```python
from build123d import *

# Parameters (mm, degrees)
BOSS_EXTRUDE1_DEPTH         = 40
TAP_DRILL_FOR_M6X1_0_TAP1_D = 5
TAP_DRILL_FOR_M6X1_0_TAP2_D = 5


with BuildPart() as part:
    # Sketch1 → Boss-Extrude1 (new body)
    with BuildSketch(Plane.XY):
        Polygon((0, 0), (0, -30), (32, -30), (32, -28), (2, -28), (2, 0), align=None)
    extrude(amount=BOSS_EXTRUDE1_DEPTH)

    # Tap Drill for M6x1.0 Tap1 (through all)
    with Locations(Plane(origin=(0, -28, 0), x_dir=(1, 0, 0), z_dir=(0, 1, 0))):
        with Locations((14.5, -7.5), (14.5, -32.5)):
            Hole(TAP_DRILL_FOR_M6X1_0_TAP1_D / 2)

    # Tap Drill for M6x1.0 Tap2 (through all)
    with Locations(Plane(origin=(2, 0, 0), x_dir=(0, 0, -1), z_dir=(1, 0, 0))):
        with Locations((-32, -14), (-8, -14)):
            Hole(TAP_DRILL_FOR_M6X1_0_TAP2_D / 2)


solid = part.part
```
Here's how the part is built. I have some questions about the finished solid (model axes, mm). A direction names the side the tool comes from. Round coordinates to 2 decimals unless told otherwise and drop trailing zeros. Order: outer loops, then holes, each group sorted by start corner. A loop starts at its lowest first (then second) coordinate and runs counter-clockwise, first axis right, second up. Notation, with made-up numbers: (29.25, 29.25) -> (59.25, 29.25) arc R17 ccw to (59.25, 38.25) -> close; hole circle Ø9 at (-12.75, -3). An arc over 180 degrees is marked (long way). Use a Markdown table: item, result. Add a question column.
(1) If we mould it in two halves opening along Z, with no side actions, what happens to faces 3 (the face through (17, -28, 20)), 4 (the face through (16.5, -29, 9)), 5 (the face through (8.8, -28.3, 40))? For each: released by +Z, released by -Z, zero draft, split by the parting line, or undercut.
(2) Suppose I cut it at D-D, the plane z = 3. Please give me the cut outline in (x, y), and give its area (3 significant figures).
(3) For faces 1 (the face through (16.34, -29.01, 30.81)), 2 (the face through (2, -14, 20)), which set-ups out of +Z, -Z, +X, -X, +Y, -Y let a thin tool reach every point of the face, with its end or its side?
(4) Suppose I cut it at A-A, the plane y = -14. Please give me the cut outline in (x, z).
(5) Suppose I cut it at C-C, the plane z = 32. Please give me the cut outline in (x, y).
(6) For pin 1 Ø1.5 at (y, z) = (-16.5, 10) entering from +X; pin 2 Ø1 at (x, z) = (24.5, 12.5) entering from +Y; pin 3 Ø6 at (y, z) = (-13, 18.5) entering from -X; pin 4 Ø4.5 at (x, z) = (14.5, 7.5) entering from +Y, each with a flat end and sliding along its axis, tell me the tip position at first contact or that it passes through.
(7) Suppose I cut it at B-B, the plane x = 16. Please give me the cut outline in (y, z), and give its area (3 significant figures).
(8) I need wall thicknesses on line 1 along Z through (x, y) = (14.5, -29.2); line 2 along X through (y, z) = (-29.55, 32.5); line 3 along X through (y, z) = (-5, 15). Which ranges of each line are inside material? Lowest first, please.
Verdict:
| question | item | result |
|---|---|---|
| 1 | face 3 | zero draft |
| 1 | face 4 | undercut |
| 1 | face 5 | released by +Z |
| 2 | outline | (0, -30) -> (32, -30) -> (32, -28) -> (2, -28) -> (2, 0) -> (0, 0) -> close |
| 2 | area | 120 mm2 |
| 3 | face 1 | +Y, -Y |
| 3 | face 2 | +Z, -Z, +X, +Y |
| 4 | outline | (0, 0) -> (2, 0) -> (2, 5.5) -> (0, 5.5) -> close; (0, 10.5) -> (2, 10.5) -> (2, 29.5) -> (0, 29.5) -> close; (0, 34.5) -> (2, 34.5) -> (2, 40) -> (0, 40) -> close |
| 5 | outline | (0, -30) -> (12.05, -30) -> (12.05, -28) -> (2, -28) -> (2, -16.5) -> (0, -16.5) -> close; (0, -11.5) -> (2, -11.5) -> (2, 0) -> (0, 0) -> close; (16.95, -30) -> (32, -30) -> (32, -28) -> (16.95, -28) -> close |
| 6 | pin 1 | x = 2 |
| 6 | pin 2 | y = -28 |
| 6 | pin 3 | x = 0 |
| 6 | pin 4 | through |
| 7 | outline | (-30, 0) -> (-28, 0) -> (-28, 5.5) -> (-30, 5.5) -> close; (-30, 9.5) -> (-28, 9.5) -> (-28, 30.5) -> (-30, 30.5) -> close; (-30, 34.5) -> (-28, 34.5) -> (-28, 40) -> (-30, 40) -> close |
| 7 | area | 64.0 mm2 |
| 8 | line 1 | 0 to 5, 10 to 30, 35 to 40 |
| 8 | line 2 | 0 to 12, 17 to 32 |
| 8 | line 3 | 0 to 2 |
